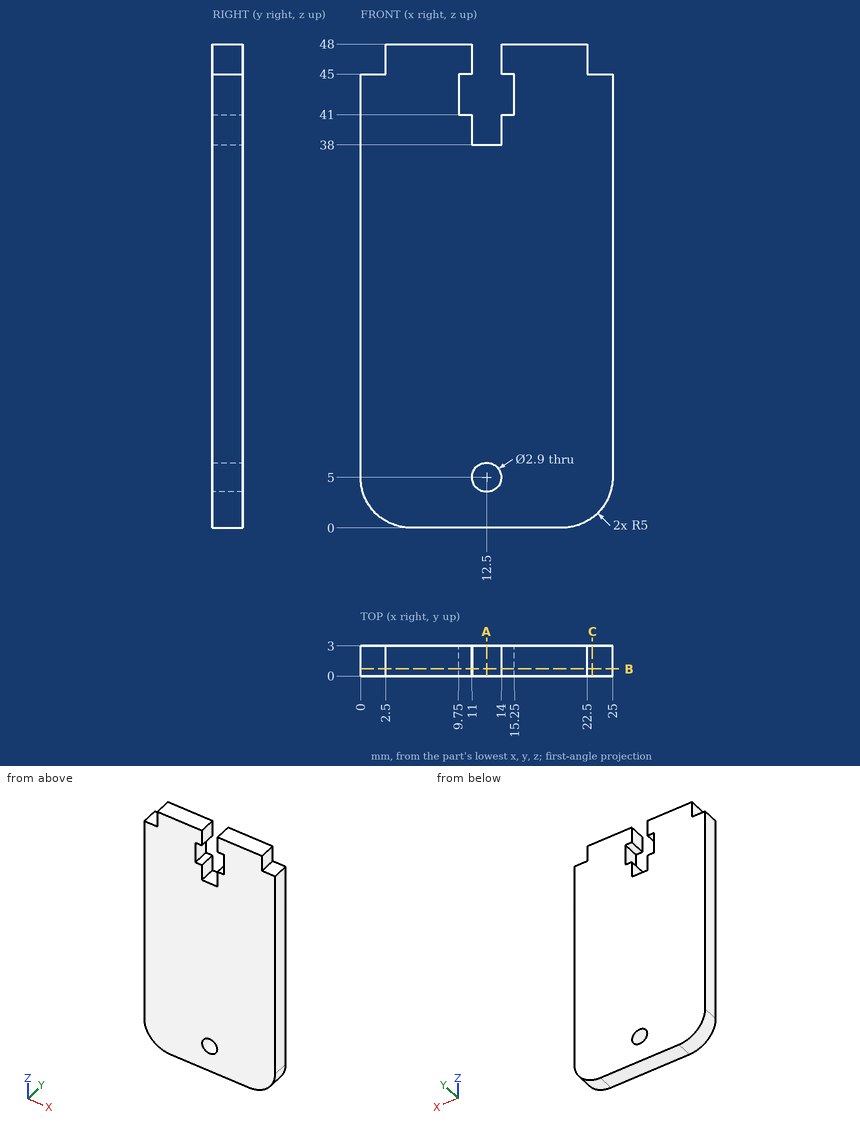
Can you work these out from the drawing? Everything is in mm from the part's minimum corner. Give positions to 0.01 mm unless a question says otherwise; leave off trailing zeros. Order: outer loops, then holes, each group sorted by start corner. A loop starts at its lowest first (then second) coordinate and runs counter-clockwise, first axis right, second up. Notation, with made-up numbers: M 38,52.25 L 80,52.25 A25 ccw 80,75.25 Z; hole C 74.25,-33 d1. An arc over 180 degrees is marked long. Use a Markdown table: item, result. Add a question column.
Item 1: Suppose I cut it at A-A (x = 12.5). List the corners of the cut face in (y, z) for me.
Item 2: Suppose I cut it at C-C (x = 23). List the corners of the cut face in (y, z) for me, then the cut area to 3 significant figures.
Item 3: If I drill on L1, parallel to X at y = 0.35, z = 44.5; L2, parallel to X at y = 0.4, z = 5.5; L3, parallel to Z at x = 3.75, y = 2.65, over which ranges is the centre line in solid material (lowest first)? Write a range as [from, to].
Item 4: Will these pins go through, and if not, where does the flat tip stop? pin 1 (0.9 mm diameter, centred on y = 2, z = 39, fed in from -X); pin 2 (0.9 mm diameter, centred on y = 1, z = 46.5, fed in from +X); pin 3 (1.5 mm diameter, centred on y = 2, z = 46.5, fed in from -X).
Item 5: Suppose I cut it at B-B (y = 0.7). List the corners of the cut face in (x, z) for me.
Answer sheet:
| question | item | result |
|---|---|---|
| 1 | outline | M 0,0 L 3,0 L 3,3.55 L 0,3.55 Z; M 0,6.45 L 3,6.45 L 3,38 L 0,38 Z |
| 2 | outline | M 0,1 L 3,1 L 3,45 L 0,45 Z |
| 2 | area | 132 mm² |
| 3 | L1 | x = [0, 9.75], [15.25, 25] |
| 3 | L2 | x = [0, 11.14], [13.86, 25] |
| 3 | L3 | z = [0.16, 48] |
| 4 | pin 1 | stops at x = 0 |
| 4 | pin 2 | stops at x = 22.5 |
| 4 | pin 3 | stops at x = 2.5 |
| 5 | outline | M 0,5 A5 ccw 5,0 L 20,0 A5 ccw 25,5 L 25,45 L 22.5,45 L 22.5,48 L 14,48 L 14,45 L 15.25,45 L 15.25,41 L 14,41 L 14,38 L 11,38 L 11,41 L 9.75,41 L 9.75,45 L 11,45 L 11,48 L 2.5,48 L 2.5,45 L 0,45 Z; hole C 12.5,5 d2.9 |
